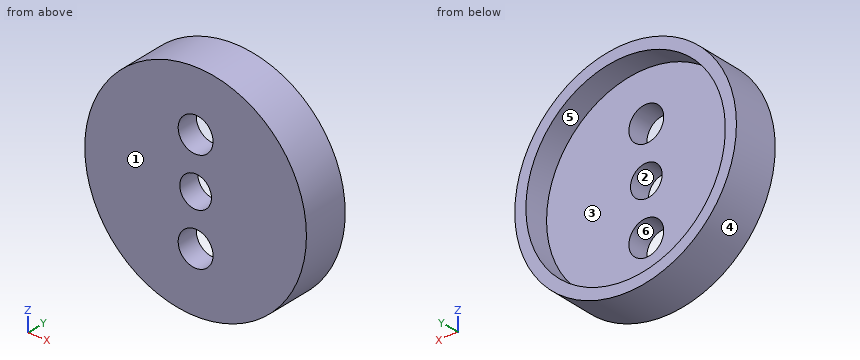
```python
from build123d import *

# Parameters (mm, degrees)
SKETCH4_R        = 17.5
SKETCH4_R_2      = 2.75
SKETCH4_R_3      = 2.5
LIDBASE_DEPTH    = 7.5
SKETCH5_R        = 15.75
LIDGROOVES_DEPTH = 4


with BuildPart() as part:
    # Sketch4 → LidBase (new body)
    with BuildSketch(Plane(origin=(0, 0, 0), x_dir=(1, 0, 0), z_dir=(0, 1, 0))):
        Circle(SKETCH4_R)
        with Locations((0, -8)):
            Circle(SKETCH4_R_2, mode=Mode.SUBTRACT)
        with Locations((0, 8)):
            Circle(SKETCH4_R_2, mode=Mode.SUBTRACT)
        Circle(SKETCH4_R_3, mode=Mode.SUBTRACT)
    extrude(amount=LIDBASE_DEPTH)

    # Sketch5 → LidGrooves (cut)
    with BuildSketch(Plane(origin=(0, 7.5, 0), x_dir=(1, 0, 0), z_dir=(0, 1, 0))):
        Circle(SKETCH5_R)
    extrude(amount=-LIDGROOVES_DEPTH, mode=Mode.SUBTRACT)


solid = part.part
```
Could you check a few things on this model? Use its own coordinates, in mm. Face numbers are marked on the shaded views. A direction names the side the tool comes from. Round coordinates to 2 decimals unless told otherwise and drop trailing zeros. Write each loop counter-clockwise with the first axis right and the second up, starting at its lowest first coordinate (ties: lowest second). Pieces come first, ordered by that corner, then holes. Notation, with made-up numbers: M 89.5,-26.5 L 131.5,-26.5 A8 ccw 131.5,-18.5 Z; hole C 3.25,37 d10. An arc over 180 degrees is marked long. Answer in a Markdown table with one row per item. Add a question column.
Q1. Imagine slicing it at B-B (z = 0). Please give me the cut outline in (x, y).
Q2. Imagine slicing it at A-A (x = 0). Please give me the cut outline in (y, z).
Q3. If I drill on line 1 (Z direction, x = 0, y = 6); line 2 (X direction, y = 1.8, z = 0); line 3 (Z direction, x = 0, y = 2.8), over which ranges is the centre line in solid material (lowest first)? Write a range as from..to.
Q4. Will these pins go through, and if not, where does the flat tip stop? pin 1 Ø16 at (x, z) = (4.5, -4.5) entering from +Y; pin 2 Ø1 at (x, y) = (2.5, 6) entering from +Z; pin 3 Ø3 at (y, z) = (6, 9.5) entering from +X.
Q5. Imagine slicing it at C-C (y = 6). Please give me the cut outline in (x, z).
Q6. Imagine slicing it at D-D (x = 8). Please give me the cut outline in (y, z).
Q7. On a 3-axis mill with a long thin cutter (end or side, diameter ignored), from which of +Z, -Z, +X, -X, +Y, -Y can I reach the whole of each face in a straight line? I mean the marked faces 5 and 6. Say none if no direction works.
Q8. If we mould it in two halves opening along X, with no side actions, what happens to the marked faces 1, 2, 3 and 4? For each: +X half, -X half, draft (parallel to the pull), parting line (faces both ways), or undercut.
Values:
| question | item | result |
|---|---|---|
| 1 | outline | M -17.5,0 L -2.5,0 L -2.5,3.5 L -15.75,3.5 L -15.75,7.5 L -17.5,7.5 Z; M 2.5,0 L 17.5,0 L 17.5,7.5 L 15.75,7.5 L 15.75,3.5 L 2.5,3.5 Z |
| 2 | outline | M 0,-17.5 L 7.5,-17.5 L 7.5,-15.75 L 3.5,-15.75 L 3.5,-10.75 L 0,-10.75 Z; M 0,-5.25 L 3.5,-5.25 L 3.5,-2.5 L 0,-2.5 Z; M 0,2.5 L 3.5,2.5 L 3.5,5.25 L 0,5.25 Z; M 0,10.75 L 3.5,10.75 L 3.5,15.75 L 7.5,15.75 L 7.5,17.5 L 0,17.5 Z |
| 3 | line 1 | -17.5..-15.75, 15.75..17.5 |
| 3 | line 2 | -17.5..-2.5, 2.5..17.5 |
| 3 | line 3 | -17.5..-10.75, -5.25..-2.5, 2.5..5.25, 10.75..17.5 |
| 4 | pin 1 | y = 3.5 |
| 4 | pin 2 | z = 17.39 |
| 4 | pin 3 | x = 15.56 |
| 5 | outline | C 0,0 d35; hole C 0,0 d31.5 |
| 6 | outline | M 0,-15.56 L 7.5,-15.56 L 7.5,-13.57 L 3.5,-13.57 L 3.5,13.57 L 7.5,13.57 L 7.5,15.56 L 0,15.56 Z |
| 7 | face 5 | +Y |
| 7 | face 6 | +Y, -Y |
| 8 | face 1 | draft |
| 8 | face 2 | undercut |
| 8 | face 3 | undercut |
| 8 | face 4 | parting line |
